Geometry check sheet. Reference: the model listing, model coordinates, mm. A direction names the side the tool comes from. Coordinates: 2 decimals unless noted, no trailing zeros. Loops run counter-clockwise (first coordinate to the right, second up) from the corner with the lowest first, then second, coordinate; pieces in that order, holes last.
from build123d import *

# Parameters (mm, degrees)
PAD_DEPTH       = 3
SKETCH001_W     = 20
SKETCH001_H     = 3
SKETCH001_W_2   = 29
POCKET_DEPTH    = 3.001
SKETCH002_W     = 3
SKETCH002_H     = 10
POCKET001_DEPTH = 328.786205


with BuildPart() as part:
    # Sketch → Pad (new body)
    with BuildSketch(Plane.XZ):
        with BuildLine():
            Line((-77.5, -25), (77.5, -25))
            Line((77.5, -25), (77.5, 25))
            Line((77.5, 25), (25, 25))
            Line((25, 25), (25, 13))
            ThreePointArc((22, 10), (24.12132, 10.87868), (25, 13))
            Line((22, 10), (-22, 10))
            ThreePointArc((-25, 13), (-24.12132, 10.87868), (-22, 10))
            Line((-25, 13), (-25, 25))
            Line((-25, 25), (-77.5, 25))
            Line((-77.5, 25), (-77.5, -25))
        make_face()
    extrude(amount=PAD_DEPTH)

    # Sketch001 (on Face12 of Pad) → Pocket (cut, through all)
    with BuildSketch(Plane.XZ.offset(3)):
        with Locations((-64.5, -18.5)):
            Rectangle(SKETCH001_W, SKETCH001_H)
        with Locations((-24.5, -18.5)):
            Rectangle(SKETCH001_W, SKETCH001_H)
        with Locations((15.5, -18.5)):
            Rectangle(SKETCH001_W, SKETCH001_H)
        with Locations((60, -18.5)):
            Rectangle(SKETCH001_W_2, SKETCH001_H)
    extrude(amount=-POCKET_DEPTH, mode=Mode.SUBTRACT)

    # Sketch002 (on Face5 of Pocket) → Pocket001 (cut, through all)
    with BuildSketch(Plane.XZ.offset(3)):
        with Locations((-76, 10)):
            Rectangle(SKETCH002_W, SKETCH002_H)
        with Locations((-76, -10)):
            Rectangle(SKETCH002_W, SKETCH002_H)
    pocket001 = extrude(amount=-POCKET001_DEPTH, mode=Mode.SUBTRACT)

    # Mirrored: Pocket001 across Sketch002 V_Axis
    add(pocket001.mirror(Plane(origin=(0, -3, 0), x_dir=(0, -1, 0), z_dir=(1, 0, 0))), mode=Mode.SUBTRACT)


solid = part.part
1) Depth check by flat-ended pin: pin 1 (0.9 mm diameter, centred on x = 0, y = -1.5, fed in from +Z); pin 2 (0.9 mm diameter, centred on y = -2, z = 12, fed in from +X). Enter the tip coordinate at first touch or a pass-through.
Data:
pin 1: stops at z = 10
pin 2: stops at x = 74.5
2) Mould release check, pull along X, two halves, no side actions. Record for faces 4 (the flat face through (77.5, -1, -20)), 5 (the flat face through (52, -1, 25)), 6 (the flat face through (-74.5, -2, -10)), 7 (the flat face through (25.5, -2, -19)): +X half, -X half, draft (parallel to the pull), parting line (faces both ways), or undercut.
Data:
face 4: +X half
face 5: draft
face 6: -X half
face 7: undercut
3) Section check C-C on y = -2.25. Count the separate pieces of the cut face and the enclosed holes in it, and give its area (3 significant figures).
Data:
separate pieces: 1
enclosed holes: 4
area: 6,620 mm2
4) Section check A-A on x = 11.5. Record the cut outline in (y, z), and give its area (3 significant figures).
Data:
outline: (-3, -25) - (0, -25) - (0, -20) - (-3, -20) - close; (-3, -17) - (0, -17) - (0, 10) - (-3, 10) - close
area: 96.0 mm2
5) Access from +Z, -Z, +X, -X, +Y, -Y to the whole of each face (thin tool, end or side, straight path). Record for faces 1 (the cylindrical face through (-24.14, -1.48, 10.9)), 2 (the flat face through (76, -2, -15)), 3 (the flat face through (-14.5, -2, -19)).
Data:
face 1: +Z, +Y, -Y
face 2: +X, +Y, -Y
face 3: +Y, -Y
6) Section check B-B on z = 11.5. Record the cut outline in (x, y), and give its area (3 significant figures).
Data:
outline: (-74.5, -3) - (-24.6, -3) - (-24.6, 0) - (-74.5, 0) - close; (24.6, -3) - (74.5, -3) - (74.5, 0) - (24.6, 0) - close
area: 299 mm2
7) Material ranges on probe 1 along X at (y, z) = (-1.45, 13); probe 2 along Z at (x, y) = (66, -1.05); probe 3 along X at (y, z) = (-1, 16.5), recorded low to high.
Data:
probe 1: x = -74.5 to -25, 25 to 74.5
probe 2: z = -25 to -20, -17 to 25
probe 3: x = -77.5 to -25, 25 to 77.5
